```python
from build123d import *

# Parameters (mm, degrees)
BASE_EXTRUDE_DEPTH = 12.7
CIRPATTERN1_COUNT  = 2
CIRPATTERN1_ANGLE  = 90
CIRPATTERN2_COUNT  = 2
CIRPATTERN2_ANGLE  = 90


with BuildPart() as part:
    # Sketch1 → Base-Extrude (new, symmetric)
    with BuildSketch(Plane.XY):
        with BuildLine():
            Line((0, 36.5125), (0, 2.6924))
            ThreePointArc((0, 2.6924), (0.788585702, 0.788585702), (2.6924, 0))
            Line((2.6924, 0), (38.5826, 0))
            ThreePointArc((38.5826, 0), (40.486414298, 0.788585702), (41.275, 2.6924))
            Line((41.275, 2.6924), (41.275, 36.5125))
            ThreePointArc((41.275, 36.5125), (36.5125, 41.275), (31.75, 36.5125))
            Line((31.75, 36.5125), (31.75, 35.47745))
            ThreePointArc((31.75, 35.47745), (33.0962, 34.13125), (34.4424, 35.47745))
            Line((34.4424, 35.47745), (34.4424, 36.5125))
            ThreePointArc((34.4424, 36.5125), (36.5125, 38.5826), (38.5826, 36.5125))
            Line((38.5826, 36.5125), (38.5826, 2.6924))
            Line((38.5826, 2.6924), (2.6924, 2.6924))
            Line((2.6924, 2.6924), (2.6924, 36.5125))
            ThreePointArc((2.6924, 36.5125), (4.7625, 38.5826), (6.8326, 36.5125))
            Line((6.8326, 36.5125), (6.8326, 35.47745))
            ThreePointArc((6.8326, 35.47745), (8.1788, 34.13125), (9.525, 35.47745))
            Line((9.525, 35.47745), (9.525, 36.5125))
            ThreePointArc((9.525, 36.5125), (4.7625, 41.275), (0, 36.5125))
        make_face()
    base_extrude = extrude(amount=BASE_EXTRUDE_DEPTH, both=True)

    # CirPattern1: Base-Extrude ×2 about axis
    cirpattern1_axis = Axis((0, 0, 0), (0, 0, 1))
    for i in range(1, CIRPATTERN1_COUNT):
        add(base_extrude.rotate(cirpattern1_axis, i * CIRPATTERN1_ANGLE / (CIRPATTERN1_COUNT - 1)))

    # CirPattern2: Base-Extrude ×2 about axis
    cirpattern2_axis = Axis((41.275, 0, 0), (0, 0, -1))
    for i in range(1, CIRPATTERN2_COUNT):
        add(base_extrude.rotate(cirpattern2_axis, i * CIRPATTERN2_ANGLE / (CIRPATTERN2_COUNT - 1)))


solid = part.part
```
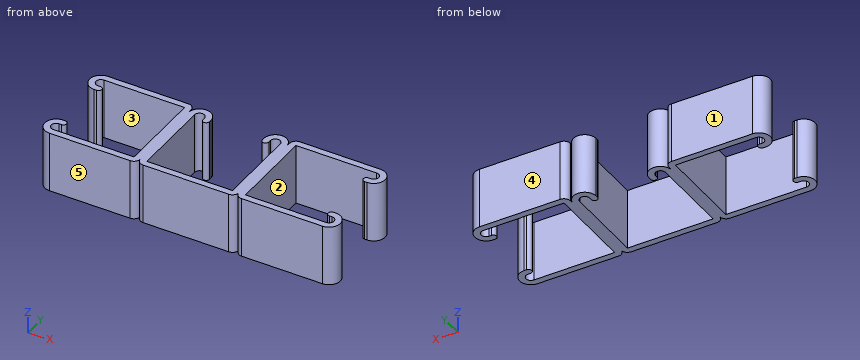
Check sheet for the modelled part. Datum: model origin and axes. Units: mm. Face numbers are marked on the shaded views. A direction names the side the tool comes from. Round coordinates to 2 decimals unless told otherwise and drop trailing zeros. Order: outer loops, then holes, each group sorted by start corner. A loop starts at its lowest first (then second) coordinate and runs counter-clockwise, first axis right, second up. Notation, with made-up numbers: (7.25, 49) -> (61.25, 49) arc R36 ccw to (61.25, 86) -> close; hole circle Ø8 at (23.5, 47). An arc over 180 degrees is marked (long way). One line per item, written item: value. Start each with the question number.
Q1. Thickness scan on line 1 (X direction, y = 4.5, z = -2.5); line 2 (X direction, y = 31, z = -4.25); line 3 (Y direction, x = 36.5, z = -7.75). Record the ranges inside material, lowest first.
Q2. Set-up check for the marked faces 1 and 2: record each of +Z, -Z, +X, -X, +Y, -Y from which the full face is reachable in a straight line by a thin tool's end or side.
Q3. Cross-section at B-B (x = -18.5). Record the boundary of the cut face in (y, z) (3 decimals).
Q4. Mould release check, pull along Y, two halves, no side actions. Record for the marked faces 3, 4 and 5: pulls with the +Y half, pulls with the -Y half, needs draft (parallel to the pull), parting line crosses it, or undercut.
Q5. Cross-section at C-C (x = 14). Record the boundary of the cut face in (y, z).
Q6. Cross-section at A-A (y = 12). Record the boundary of the cut face in (x, z).
Q7. Gauge pin test, flat ends, axial feed: pin 1 Ø2 at (x, z) = (32, 0) entering from +Y; pin 2 Ø0.8 at (y, z) = (36, 4.5) entering from +X; pin 3 Ø3 at (x, y) = (8.5, 31) entering from -Z; pin 4 Ø12.5 at (y, z) = (26, -5) entering from -X. Record the tip position at first contact, or that the pin passes through.
Completed:
1. line 1: x = -41.27 to -38.57, -2.69 to 2.69, 38.58 to 43.97, 79.84 to 82.54
1. line 2: x = -2.69 to 2.69, 38.58 to 43.97
1. line 3: y = 0 to 2.69, 38.58 to 41.27
2. face 1: +Z, -Z, +X, -X, +Y
2. face 2: +Z, -Z
3. outline: (0, -12.7) -> (2.692, -12.7) -> (2.692, 12.7) -> (0, 12.7) -> close; (38.583, -12.7) -> (41.275, -12.7) -> (41.275, 12.7) -> (38.583, 12.7) -> close
4. face 3: undercut
4. face 4: pulls with the +Y half
4. face 5: pulls with the -Y half
5. outline: (0, -12.7) -> (2.69, -12.7) -> (2.69, 12.7) -> (0, 12.7) -> close
6. outline: (-2.69, -12.7) -> (2.69, -12.7) -> (2.69, 12.7) -> (-2.69, 12.7) -> close; (38.58, -12.7) -> (43.97, -12.7) -> (43.97, 12.7) -> (38.58, 12.7) -> close
7. pin 1: stops at y = 39.73
7. pin 2: stops at x = 82.55
7. pin 3: passes through
7. pin 4: stops at x = -38.64
